Source: CAD feature listing. Evaluate the final solid. Frame: model axes, mm. Face numbers are marked on the shaded views. A direction names the side the tool comes from. Coordinates: 2 decimals unless noted, no trailing zeros. Loops run counter-clockwise (first coordinate to the right, second up) from the corner with the lowest first, then second, coordinate; pieces in that order, holes last.
Item 1: Section query A-A, the plane z = 5.2. Return the cut outline in (x, y).
Item 2: Line query: probe 1 along Z at (x, y) = (25.5, 2.6); probe 2 along X at (y, z) = (3, 12.5); probe 3 along X at (y, z) = (3.25, 1.5). Output: solid intervals per line, ascending.
Item 3: Pull-direction query (Z, two-part tool) for the marked faces 1, 2, 3 and 4; classes: +Z half, -Z half, draft (parallel to the pull), parting line (faces both ways), or undercut.
Item 4: Section query B-B, the plane y = 2.5. Return the cut outline in (x, z), then the cut area to 3 significant figures.
Item 5: Section query D-D, the plane z = 12.5. State how many separate pieces and enclosed holes the cut face has, then the cut area to 3 significant figures.
Item 6: Pin query (flat end, axial travel): pin 1 Ø0.8 at (x, z) = (15.5, 24.5) entering from +Y; pin 2 Ø1.1 at (y, z) = (5, 24.5) entering from -X; pin 3 Ø0.8 at (y, z) = (5, 24.5) entering from +X; pin 4 Ø1 at (x, z) = (5.8, 5.2) entering from -Y. Return the tip coordinate at first contact, or that it passes through.
Item 7: Reachability of the marked faces 5 and 6 from +Z, -Z, +X, -X, +Y, -Y: full face, straight path, thin tool, end or side. Return the list, or none.
Item 8: Section query C-C, the plane x = 25.5. Return the cut outline in (y, z), then the cut area to 3 significant figures.
```python
from build123d import *

# Parameters (mm, degrees)
FACE004_W          = 8.25
FACE004_H          = 1
EXTRUSION003_DEPTH = 0.2
FACE005_W          = 6.85
FACE005_H          = 1
EXTRUSION004_DEPTH = 0.2
BOX008_W           = 8.25
BOX008_H           = 2.55
BOX008_DEPTH       = 1
BOX009_W           = 6.85
BOX009_H           = 2.1
BOX009_DEPTH       = 1
BOX007_W           = 7.85
BOX007_H           = 2.1
BOX007_DEPTH       = 10
BOX006_W           = 9.25
BOX006_H           = 2.55
BOX006_DEPTH       = 10
BOX003_W           = 27
BOX003_H           = 1.5
BOX003_DEPTH       = 21
BOX002_W           = 29
BOX002_H           = 1.5
BOX002_DEPTH       = 23
CYLINDER004_R      = 0.8
CYLINDER004_DEPTH  = 20.6
CYLINDER002_R      = 1.2
CYLINDER002_DEPTH  = 10.6
CYLINDER001_R      = 1.2
CYLINDER001_DEPTH  = 10.6
CYLINDER003_R      = 2.2
CYLINDER003_DEPTH  = 2.6
BOX001_W           = 27
BOX001_H           = 2.6
BOX001_DEPTH       = 21
BOX_W              = 31
BOX_H              = 4.6
BOX_DEPTH          = 25
CYLINDER_R         = 2.2
CYLINDER_DEPTH     = 2.6
CYLINDER005_R      = 1.5
CYLINDER005_DEPTH  = 2.6
BOX005_W           = 29
BOX005_H           = 0.45
BOX005_DEPTH       = 23
BOX004_W           = 31
BOX004_H           = 0.45
BOX004_DEPTH       = 25
FILLET_R           = 2
CHAMFER_SIZE       = 1
FACE001_R          = 2.2
FACE001_R_2        = 1.2
EXTRUSION001_DEPTH = 0.2
FACE003_R          = 1.5
FACE003_R_2        = 0.8
EXTRUSION002_DEPTH = 0.2
FACE_R             = 2.2
FACE_R_2           = 1.2
EXTRUSION_DEPTH    = 0.2


with BuildPart() as extrusion003:
    # Face004 → Extrusion003 (new body)
    with BuildSketch(Plane(origin=(21.995, 6.3, 24.5), x_dir=(1, 0, 0), z_dir=(0, 1, 0))):
        Rectangle(FACE004_W, FACE004_H)
    extrude(amount=EXTRUSION003_DEPTH)


with BuildPart() as extrusion004:
    # Face005 → Extrusion004 (new body)
    with BuildSketch(Plane(origin=(8.995, 6.05, 24.5), x_dir=(1, 0, 0), z_dir=(0, 1, 0))):
        Rectangle(FACE005_W, FACE005_H)
    extrude(amount=EXTRUSION004_DEPTH)


with BuildPart() as obj1:
    # Box008 → Box008 (new body)
    with BuildSketch(Plane(origin=(17.87, 3.75, 24), x_dir=(1, 0, 0), z_dir=(0, 0, 1))):
        with Locations((4.125, 1.275)):
            Rectangle(BOX008_W, BOX008_H)
    extrude(amount=BOX008_DEPTH)


with BuildPart() as micro_cutoff:
    # Box009 → Box009 (new body)
    with BuildSketch(Plane(origin=(5.57, 3.95, 24), x_dir=(1, 0, 0), z_dir=(0, 0, 1))):
        with Locations((3.425, 1.05)):
            Rectangle(BOX009_W, BOX009_H)
    extrude(amount=BOX009_DEPTH)


with BuildPart() as countersunkleft:
    # Cone → Cone (revolve)
    with BuildSketch(Plane(origin=(5.5, 0, 12.5), x_dir=(1, 0, 0), z_dir=(0, 0, 1))):
        Polygon((0, 0), (2.25, 0), (1.2, 1.5), (0, 1.5), align=None)
    revolve(axis=Axis((5.5, 0, 12.5), (0, 1, 0)))


with BuildPart() as countersunk:
    # Cone001 → Cone001 (revolve)
    with BuildSketch(Plane(origin=(25.5, 0, 12.5), x_dir=(1, 0, 0), z_dir=(0, 0, 1))):
        Polygon((0, 0), (2.25, 0), (1.2, 1.5), (0, 1.5), align=None)
    revolve(axis=Axis((25.5, 0, 12.5), (0, 1, 0)))

    # Fusion005: union counterSunkLeft
    add(countersunkleft.part)


with BuildPart() as micro_cutout:
    # Box007 → Box007 (new body)
    with BuildSketch(Plane(origin=(5.07, 3.95, 20), x_dir=(1, 0, 0), z_dir=(0, 0, 1))):
        with Locations((3.925, 1.05)):
            Rectangle(BOX007_W, BOX007_H)
    extrude(amount=BOX007_DEPTH)


with BuildPart() as connector_cutouts:
    # Box006 → Box006 (new body)
    with BuildSketch(Plane(origin=(17.37, 3.75, 19), x_dir=(1, 0, 0), z_dir=(0, 0, 1))):
        with Locations((4.625, 1.275)):
            Rectangle(BOX006_W, BOX006_H)
    extrude(amount=BOX006_DEPTH)

    # Fusion006: union Micro_cutout
    add(micro_cutout.part)


with BuildPart() as cube001:
    # Box003 → Box003 (new body)
    with BuildSketch(Plane(origin=(2, 3.1, 2), x_dir=(1, 0, 0), z_dir=(0, 0, 1))):
        with Locations((13.5, 0.75)):
            Rectangle(BOX003_W, BOX003_H)
    extrude(amount=BOX003_DEPTH)


with BuildPart() as cut004:
    # Box002 → Box002 (new body)
    with BuildSketch(Plane(origin=(1, 3.1, 1), x_dir=(1, 0, 0), z_dir=(0, 0, 1))):
        with Locations((14.5, 0.75)):
            Rectangle(BOX002_W, BOX002_H)
    extrude(amount=BOX002_DEPTH)

    # Cut004: cut Cube001
    add(cube001.part, mode=Mode.SUBTRACT)


with BuildPart() as obj2:
    # Cylinder004 → Cylinder004 (new body)
    with BuildSketch(Plane(origin=(5.8, 12, 5.2), x_dir=(1, 0, 0), z_dir=(0, -1, 0))):
        Circle(CYLINDER004_R)
    extrude(amount=CYLINDER004_DEPTH)


with BuildPart() as pcbholderhole001:
    # Cylinder002 → Cylinder002 (new body)
    with BuildSketch(Plane(origin=(5.5, 4.6, 12.5), x_dir=(1, 0, 0), z_dir=(0, -1, 0))):
        Circle(CYLINDER002_R)
    extrude(amount=CYLINDER002_DEPTH)


with BuildPart() as pcbholes:
    # Cylinder001 → Cylinder001 (new body)
    with BuildSketch(Plane(origin=(25.5, 4.6, 12.5), x_dir=(1, 0, 0), z_dir=(0, -1, 0))):
        Circle(CYLINDER001_R)
    extrude(amount=CYLINDER001_DEPTH)

    # Fusion001: union pcbHolderHole001
    add(pcbholderhole001.part)


with BuildPart() as pcbholder001:
    # Cylinder003 → Cylinder003 (new body)
    with BuildSketch(Plane(origin=(5.5, 4.6, 12.5), x_dir=(1, 0, 0), z_dir=(0, -1, 0))):
        Circle(CYLINDER003_R)
    extrude(amount=CYLINDER003_DEPTH)


with BuildPart() as innercut:
    # Box001 → Box001 (new body)
    with BuildSketch(Plane(origin=(2, 2, 2), x_dir=(1, 0, 0), z_dir=(0, 0, 1))):
        with Locations((13.5, 1.3)):
            Rectangle(BOX001_W, BOX001_H)
    extrude(amount=BOX001_DEPTH)


with BuildPart() as cut:
    # Box → Box (new body)
    with BuildSketch(Plane.XY):
        with Locations((15.5, 2.3)):
            Rectangle(BOX_W, BOX_H)
    extrude(amount=BOX_DEPTH)

    # Cut: cut innerCut
    add(innercut.part, mode=Mode.SUBTRACT)


with BuildPart() as obj3:
    # Cylinder → Cylinder (new body)
    with BuildSketch(Plane(origin=(25.5, 4.6, 12.5), x_dir=(1, 0, 0), z_dir=(0, -1, 0))):
        Circle(CYLINDER_R)
    extrude(amount=CYLINDER_DEPTH)

    # Fusion: union pcbHolder001, Cut
    add(pcbholder001.part)
    add(cut.part)

    # Cut001: cut pcbHoles
    add(pcbholes.part, mode=Mode.SUBTRACT)


with BuildPart() as cut009:
    # Cylinder005 → Cylinder005 (new body)
    with BuildSketch(Plane(origin=(5.8, 4.6, 5.2), x_dir=(1, 0, 0), z_dir=(0, -1, 0))):
        Circle(CYLINDER005_R)
    extrude(amount=CYLINDER005_DEPTH)

    # Fusion002: union obj3
    add(obj3.part)

    # Cut002: cut obj2
    add(obj2.part, mode=Mode.SUBTRACT)

    # Cut009: cut Cut004
    add(cut004.part, mode=Mode.SUBTRACT)


with BuildPart() as cube003:
    # Box005 → Box005 (new body)
    with BuildSketch(Plane(origin=(1, 4.6, 1), x_dir=(1, 0, 0), z_dir=(0, 0, 1))):
        with Locations((14.5, 0.225)):
            Rectangle(BOX005_W, BOX005_H)
    extrude(amount=BOX005_DEPTH)


with BuildPart() as chamfer_body:
    # Box004 → Box004 (new body)
    with BuildSketch(Plane(origin=(0, 4.6, 0), x_dir=(1, 0, 0), z_dir=(0, 0, 1))):
        with Locations((15.5, 0.225)):
            Rectangle(BOX004_W, BOX004_H)
    extrude(amount=BOX004_DEPTH)

    # Cut006: cut Cube003
    add(cube003.part, mode=Mode.SUBTRACT)

    # Fusion004: union Cut009
    add(cut009.part)

    # Cut010: cut connector_cutouts
    add(connector_cutouts.part, mode=Mode.SUBTRACT)

    # Cut011: cut counterSunk
    add(countersunk.part, mode=Mode.SUBTRACT)

    # Fusion007: union obj1, Micro_cutoff
    add(obj1.part)
    add(micro_cutoff.part)

    # Fillet
    fillet_edges = [chamfer_body.edges().sort_by_distance(p)[0] for p in [
        (0, 0, 12.5),
        (31, 0, 12.5),
    ]]
    fillet(fillet_edges, radius=FILLET_R)

    # Chamfer
    chamfer_edges = [chamfer_body.edges().sort_by_distance(p)[0] for p in [
        (0, 3.3, 25),
        (0, 3.3, 0),
        (0.585786, 0.585786, 25),
        (15.5, 0, 25),
        (30.414214, 0.585786, 25),
        (31, 3.3, 25),
        (0.585786, 0.585786, 0),
        (0, 4.825, 25),
        (0, 4.825, 0),
        (15.5, 0, 0),
        (31, 3.3, 0),
        (30.414214, 0.585786, 0),
        (31, 4.825, 25),
        (31, 4.825, 0),
    ]]
    chamfer(chamfer_edges, length=CHAMFER_SIZE)


with BuildPart() as extrusion001:
    # Face001 → Extrusion001 (new body)
    with BuildSketch(Plane(origin=(5.5, 4.6, 12.5), x_dir=(1, 0, 0), z_dir=(0, 1, 0))):
        Circle(FACE001_R)
        Circle(FACE001_R_2, mode=Mode.SUBTRACT)
    extrude(amount=EXTRUSION001_DEPTH)


with BuildPart() as extrusion002:
    # Face003 → Extrusion002 (new body)
    with BuildSketch(Plane(origin=(5.8, 4.6, 5.2), x_dir=(1, 0, 0), z_dir=(0, 1, 0))):
        Circle(FACE003_R)
        Circle(FACE003_R_2, mode=Mode.SUBTRACT)
    extrude(amount=EXTRUSION002_DEPTH)


with BuildPart() as fusion010:
    # Face → Extrusion (new body)
    with BuildSketch(Plane(origin=(25.5, 4.6, 12.5), x_dir=(1, 0, 0), z_dir=(0, 1, 0))):
        Circle(FACE_R)
        Circle(FACE_R_2, mode=Mode.SUBTRACT)
    extrude(amount=EXTRUSION_DEPTH)

    # Fusion008: union Extrusion001, Extrusion002
    add(extrusion001.part)
    add(extrusion002.part)

    # Fusion009: union Chamfer body
    add(chamfer_body.part)

    # Fusion010: union Extrusion003, Extrusion004
    add(extrusion003.part)
    add(extrusion004.part)


solid = fusion010.part
```
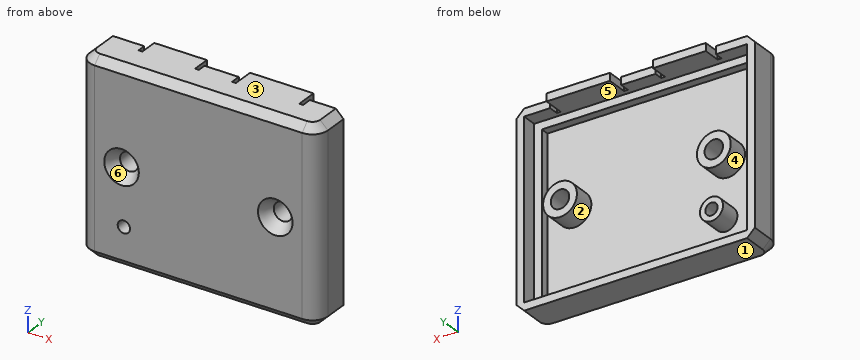
Verdict:
1. outline: (0, 2) arc R2 ccw to (2, 0) - (5, 0) - (5, 4.8) - (4.3, 4.8) - (4.3, 2) - (2, 2) - (2, 3.1) - (1, 3.1) - (1, 5.05) - (0, 5.05) - close; (6.6, 0) - (29, 0) arc R2 ccw to (31, 2) - (31, 5.05) - (30, 5.05) - (30, 3.1) - (29, 3.1) - (29, 2) - (7.3, 2) - (7.3, 4.8) - (6.6, 4.8) - close
2. probe 1: z = 0 to 2, 10.3 to 11.3, 13.7 to 14.7, 23 to 25
2. probe 2: x = 0 to 2, 3.3 to 4.3, 6.7 to 7.7, 23.3 to 24.3, 26.7 to 27.7, 29 to 31
2. probe 3: x = 0 to 1, 30 to 31
3. face 1: -Z half
3. face 2: undercut
3. face 3: +Z half
3. face 4: undercut
4. outline: (0, 1) - (1, 0) - (30, 0) - (31, 1) - (31, 24) - (30, 25) - (1, 25) - (0, 24) - close; circle Ø4.4 at (5.5, 12.5); circle Ø3 at (5.8, 5.2); circle Ø4.4 at (25.5, 12.5); hole (2, 2) - (29, 2) - (29, 23) - (2, 23) - close; hole circle Ø2.4 at (5.5, 12.5); hole circle Ø1.6 at (5.8, 5.2); hole circle Ø2.4 at (25.5, 12.5)
4. area: 232 mm2
5. separate pieces: 3
5. enclosed holes: 0
5. area: 67.0 mm2
6. pin 1: stops at y = 5.05
6. pin 2: stops at x = 0
6. pin 3: stops at x = 30.9
6. pin 4: passes through
7. face 5: +Y
7. face 6: -Y
8. outline: (0, 1) - (1, 0) - (5.05, 0) - (5.05, 1) - (3.1, 1) - (3.1, 2) - (2, 2) - (2, 10.3) - (4.8, 10.3) - (4.8, 11.3) - (1.5, 11.3) - (0, 10.25) - close; (0, 14.75) - (1.5, 13.7) - (4.8, 13.7) - (4.8, 14.7) - (2, 14.7) - (2, 23) - (3.1, 23) - (3.1, 24) - (6.5, 24) - (6.5, 25) - (1, 25) - (0, 24) - close
8. area: 58.0 mm2
